Design review of the part built by this model. Coordinates are the model's own, in mm. A direction names the side the tool comes from. Coordinates: 2 decimals unless noted, no trailing zeros. Write each loop counter-clockwise with the first axis right and the second up, starting at its lowest first coordinate (ties: lowest second). Pieces come first, ordered by that corner, then holes. Notation, with made-up numbers: (51.25, 71) - (61.25, 71) arc R29 cw to (61.25, 93) - close; hole circle Ø5 at (78, -20.75). An arc over 180 degrees is marked (long way). Use a Markdown table: item, result.
from build123d import *

# Parameters (mm, degrees)
SKETCH_W      = 30
SKETCH_H      = 80
PAD_DEPTH     = 2
SKETCH001_R   = 2.354301
SKETCH001_R_2 = 2.478142
SKETCH001_R_3 = 2.498945
SKETCH001_W   = 5
SKETCH001_H   = 30
POCKET_DEPTH  = 5


with BuildPart() as part:
    # Sketch → Pad (new body)
    with BuildSketch(Plane.XY):
        with Locations((15, 0)):
            Rectangle(SKETCH_W, SKETCH_H)
    extrude(amount=PAD_DEPTH)

    # Sketch001 (on Face5 of Pad) → Pocket (cut)
    with BuildSketch(Plane(origin=(0, 0, 0), x_dir=(1, 0, 0), z_dir=(0, 0, -1))):
        with Locations((15, -30)):
            Circle(SKETCH001_R)
        with Locations((15, -15)):
            Circle(SKETCH001_R_2)
        with Locations((15, 15)):
            Circle(SKETCH001_R_2)
        with Locations((15, 30)):
            Circle(SKETCH001_R_3)
        with Locations((7.5, 20)):
            Rectangle(SKETCH001_W, SKETCH001_H)
        with Locations((22.5, 20)):
            Rectangle(SKETCH001_W, SKETCH001_H)
        with Locations((7.5, -20)):
            Rectangle(SKETCH001_W, SKETCH001_H)
        with Locations((22.5, -20)):
            Rectangle(SKETCH001_W, SKETCH001_H)
    extrude(amount=-POCKET_DEPTH, mode=Mode.SUBTRACT)


solid = part.part
(1) For L1, parallel to Y at x = 15, z = 0.5; L2, parallel to Y at x = 9.5, z = 1.8; L3, parallel to X at y = -26, z = 0.9, list the stretches that pass through material, from the lowest coordinate up. Write a range as from..to.
Determined:
| item | result |
|---|---|
| L1 | -40..-32.5, -27.5..-17.48, -12.52..12.52, 17.48..27.65, 32.35..40 |
| L2 | -40..-35, -5..5, 35..40 |
| L3 | 0..5, 10..20, 25..30 |
(2) Take a section at C-C on z = 1.1. State how many separate pieces and enclosed holes the cut face has, and give its area (3 significant figures).
Determined:
| item | result |
|---|---|
| separate pieces | 1 |
| enclosed holes | 8 |
| area | 1,720 mm2 |
(3) Take a section at D-D on x = 14.5. Write out the cut boundary in (y, z), and give its area (3 significant figures).
Determined:
| item | result |
|---|---|
| outline | (-40, 0) - (-32.45, 0) - (-32.45, 2) - (-40, 2) - close; (-27.55, 0) - (-17.43, 0) - (-17.43, 2) - (-27.55, 2) - close; (-12.57, 0) - (12.57, 0) - (12.57, 2) - (-12.57, 2) - close; (17.43, 0) - (27.7, 0) - (27.7, 2) - (17.43, 2) - close; (32.3, 0) - (40, 0) - (40, 2) - (32.3, 2) - close |
| area | 122 mm2 |
(4) Take a section at A-A on y = 30. Write out the cut boundary in (x, z), and give its area (3 significant figures).
Determined:
| item | result |
|---|---|
| outline | (0, 0) - (5, 0) - (5, 2) - (0, 2) - close; (10, 0) - (12.65, 0) - (12.65, 2) - (10, 2) - close; (17.35, 0) - (20, 0) - (20, 2) - (17.35, 2) - close; (25, 0) - (30, 0) - (30, 2) - (25, 2) - close |
| area | 30.6 mm2 |
(5) Take a section at B-B on y = -24. Write out the cut boundary in (x, z).
Determined:
| item | result |
|---|---|
| outline | (0, 0) - (5, 0) - (5, 2) - (0, 2) - close; (10, 0) - (20, 0) - (20, 2) - (10, 2) - close; (25, 0) - (30, 0) - (30, 2) - (25, 2) - close |
(6) Machinability: for faces 1 (the flat face through (0, -1, 1)), 2 (the flat face through (5, 20, 1)), which of the approach directions +Z, -Z, +X, -X, +Y, -Y give a long, thin tool a straight path to every point of the face, cutting with its end or side? Answer none if there is none.
Determined:
| item | result |
|---|---|
| face 1 | +Z, -Z, -X, +Y, -Y |
| face 2 | +Z, -Z |
(7) For pin 1 (4 mm diameter, centred on x = 15, y = -15, fed in from +Z), flat-tipped, find the tip position at first contact; note if it passes through.
Determined:
| item | result |
|---|---|
| pin 1 | through |
(8) Draft analysis for pull direction Y (two halves, no side actions). For faces 3 (the flat face through (7, 35, 1)), 4 (the flat face through (30, -1, 1)), 5 (the flat face through (15, -40, 1)), state which applies: +Y half, -Y half, draft (parallel to the pull), parting line (faces both ways), or undercut.
Determined:
| item | result |
|---|---|
| face 3 | undercut |
| face 4 | draft |
| face 5 | -Y half |
